from build123d import *

# Parameters (mm, degrees)
AUFSATZ_LINEAR_AUSTRAGEN1_DEPTH      = 43
AUFSATZ_LINEAR_AUSTRAGEN2_DEPTH      = 5
SCHNITT_LINEAR_AUSTRAGEN1_REACH      = 157.451
SKIZZE3_R                            = 1.5
SKIZZE4_W                            = 8
SKIZZE4_H                            = 16
SCHNITT_LINEAR_AUSTRAGEN2_DEPTH      = 18
SKIZZE5_W                            = 30
SKIZZE5_H                            = 39
SCHNITT_LINEAR_AUSTRAGEN3_DEPTH      = 18
SKIZZE6_W                            = 7
SKIZZE6_H                            = 7.5
SKIZZE6_H_2                          = 14
SKIZZE6_H_3                          = 5.5
AUFSATZ_LINEAR_AUSTRAGEN3_DEPTH      = 4
VERRUNDUNG1_R                        = 2
F_3_4_3_4_DURCHMESSER_BOHRUNG1_D     = 3.4
F_3_4_3_4_DURCHMESSER_BOHRUNG1_DEPTH = 4
SKIZZE10_W                           = 10
SKIZZE10_H                           = 33
SCHNITT_LINEAR_AUSTRAGEN4_DEPTH      = 1
SKIZZE11_W                           = 10
SKIZZE11_H                           = 33
SCHNITT_LINEAR_AUSTRAGEN5_DEPTH      = 0.1
SCHNITT_LINEAR_AUSTRAGEN7_DEPTH      = 39
SKIZZE15_W                           = 10.432594073
SKIZZE15_H                           = 24
SCHNITT_LINEAR_AUSTRAGEN10_DEPTH     = 16
SKIZZE16_W                           = 2.1
SKIZZE16_H                           = 39
SCHNITT_LINEAR_AUSTRAGEN11_DEPTH     = 2
VERRUNDUNG2_R                        = 20
VERRUNDUNG3_R                        = 10
SKIZZE17_W                           = 6
SKIZZE17_H                           = 6
AUFSATZ_LINEAR_AUSTRAGEN4_DEPTH      = 5
FASE1_SIZE                           = 6
F_3_4_3_4_DURCHMESSER_BOHRUNG2_D     = 3.4
F_3_4_3_4_DURCHMESSER_BOHRUNG2_DEPTH = 5
F_3_4_3_4_DURCHMESSER_BOHRUNG2_TIP   = 1.021463052


with BuildPart() as part:
    # Skizze1 → Aufsatz-Linear austragen1 (new body)
    with BuildSketch(Plane(origin=(0, 0, 0), x_dir=(1, 0, 0), z_dir=(0, 1, 0))):
        Polygon((0, 0), (50, 0), (78.641941074, 13.355956467), (70.189575839, 31.482112208), (34.843572145, 15), (0, 15), align=None)
    extrude(amount=AUFSATZ_LINEAR_AUSTRAGEN1_DEPTH)

    # Skizze2 → Aufsatz-Linear austragen2 (add)
    with BuildSketch(Plane(origin=(69.711631316, 0, -32.507067545), x_dir=(-0.4226182617407004, 0, -0.9063077870366495), z_dir=(0.9063077870366495, 0, -0.4226182617407004))):
        Polygon((-21.130913087, 43), (8.869086913, 43), (54.544231126, 88.675144213), (68.686366749, 74.533008589), (15.65335816, 21.5), (68.686366749, -31.533008589), (54.544231126, -45.675144213), (8.869086913, 0), (-21.130913087, 0), align=None)
    extrude(amount=AUFSATZ_LINEAR_AUSTRAGEN2_DEPTH)

    # Skizze3 → Schnitt-Linear austragen1 (cut, up to next)
    with BuildSketch(Plane.XY, mode=Mode.PRIVATE) as schnitt_linear_austragen1_sk1:
        with Locations((6, 39)):
            Circle(SKIZZE3_R)
    schnitt_linear_austragen1_tool1 = extrude(schnitt_linear_austragen1_sk1.sketch, amount=-SCHNITT_LINEAR_AUSTRAGEN1_REACH, mode=Mode.PRIVATE) & part.part
    # Skizze3 → Schnitt-Linear austragen1 (cut, up to next)
    with BuildSketch(Plane.XY, mode=Mode.PRIVATE) as schnitt_linear_austragen1_sk2:
        with Locations((20, 39)):
            Circle(SKIZZE3_R)
    schnitt_linear_austragen1_tool2 = extrude(schnitt_linear_austragen1_sk2.sketch, amount=-SCHNITT_LINEAR_AUSTRAGEN1_REACH, mode=Mode.PRIVATE) & part.part
    # Skizze3 → Schnitt-Linear austragen1 (cut, up to next)
    with BuildSketch(Plane.XY, mode=Mode.PRIVATE) as schnitt_linear_austragen1_sk3:
        with Locations((6, 4)):
            Circle(SKIZZE3_R)
    schnitt_linear_austragen1_tool3 = extrude(schnitt_linear_austragen1_sk3.sketch, amount=-SCHNITT_LINEAR_AUSTRAGEN1_REACH, mode=Mode.PRIVATE) & part.part
    # Skizze3 → Schnitt-Linear austragen1 (cut, up to next)
    with BuildSketch(Plane.XY, mode=Mode.PRIVATE) as schnitt_linear_austragen1_sk4:
        with Locations((20, 4)):
            Circle(SKIZZE3_R)
    schnitt_linear_austragen1_tool4 = extrude(schnitt_linear_austragen1_sk4.sketch, amount=-SCHNITT_LINEAR_AUSTRAGEN1_REACH, mode=Mode.PRIVATE) & part.part
    add(schnitt_linear_austragen1_tool1.solids().sort_by_distance((6, 39, 0))[0], mode=Mode.SUBTRACT)
    add(schnitt_linear_austragen1_tool2.solids().sort_by_distance((20, 39, 0))[0], mode=Mode.SUBTRACT)
    add(schnitt_linear_austragen1_tool3.solids().sort_by_distance((6, 4, 0))[0], mode=Mode.SUBTRACT)
    add(schnitt_linear_austragen1_tool4.solids().sort_by_distance((20, 4, 0))[0], mode=Mode.SUBTRACT)

    # Skizze4 → Schnitt-Linear austragen2 (cut)
    with BuildSketch(Plane.ZY):
        with Locations((-4, 21.5)):
            Rectangle(SKIZZE4_W, SKIZZE4_H)
    extrude(amount=-SCHNITT_LINEAR_AUSTRAGEN2_DEPTH, mode=Mode.SUBTRACT)

    # Skizze5 → Schnitt-Linear austragen3 (cut)
    with BuildSketch(Plane(origin=(0.477944523, 0, 1.024955337), x_dir=(-0.9063077870366492, 0, 0.4226182617407011), z_dir=(-0.4226182617407011, 0, -0.9063077870366492))):
        with Locations((-60.918274689, 21.5)):
            Rectangle(SKIZZE5_W, SKIZZE5_H)
    extrude(amount=-SCHNITT_LINEAR_AUSTRAGEN3_DEPTH, mode=Mode.SUBTRACT)

    # Skizze6 → Aufsatz-Linear austragen3 (add)
    with BuildSketch(Plane(origin=(8.085073234, 0, 17.338495504), x_dir=(-0.9063077870366492, 0, 0.42261826174070133), z_dir=(-0.42261826174070133, 0, -0.9063077870366492))):
        with Locations((-72.418274689, 37.25)):
            Rectangle(SKIZZE6_W, SKIZZE6_H)
        with Locations((-72.418274689, 18.5)):
            Rectangle(SKIZZE6_W, SKIZZE6_H_2)
        with Locations((-72.418274689, 4.75)):
            Rectangle(SKIZZE6_W, SKIZZE6_H_3)
    extrude(amount=AUFSATZ_LINEAR_AUSTRAGEN3_DEPTH)

    # Verrundung1
    verrundung1_edges = [part.edges().sort_by_distance(p)[0] for p in [
        (69.701005731, 33.5, -13.600241521),
        (69.701005731, 11.5, -13.600241521),
        (69.701005731, 25.5, -13.600241521),
        (69.701005731, 7.5, -13.600241521),
    ]]
    fillet(verrundung1_edges, radius=VERRUNDUNG1_R)

    # Ø3.4 (3.4) Durchmesser Bohrung1
    with Locations(Plane(origin=(6.394600187, 0, 13.713264356), x_dir=(-0.906307787036649, 0, 0.4226182617407016), z_dir=(-0.4226182617407016, 0, -0.906307787036649))):
        with Locations((-72.418274689, 37), (-72.418274689, 22), (-71.418274689, 14.1), (-71.418274689, 5)):
            Hole(F_3_4_3_4_DURCHMESSER_BOHRUNG1_D / 2, depth=F_3_4_3_4_DURCHMESSER_BOHRUNG1_DEPTH)

    # Skizze10 → Schnitt-Linear austragen4 (cut)
    with BuildSketch(Plane(origin=(8.085073234, 0, 17.338495504), x_dir=(-0.9063077870366492, 0, 0.42261826174070133), z_dir=(-0.42261826174070133, 0, -0.9063077870366492))):
        with Locations((-63.918274689, 21.5)):
            Rectangle(SKIZZE10_W, SKIZZE10_H)
    extrude(amount=-SCHNITT_LINEAR_AUSTRAGEN4_DEPTH, mode=Mode.SUBTRACT)

    # Skizze11 → Schnitt-Linear austragen5 (cut)
    with BuildSketch(Plane(origin=(8.930309758, 0, 19.151111078), x_dir=(0.9063077870366492, 0, -0.42261826174070133), z_dir=(0.42261826174070133, 0, 0.9063077870366492))):
        with Locations((63.918274689, 21.5)):
            Rectangle(SKIZZE11_W, SKIZZE11_H)
    extrude(amount=-SCHNITT_LINEAR_AUSTRAGEN5_DEPTH, mode=Mode.SUBTRACT)

    # Skizze12 → Schnitt-Linear austragen7 (cut)
    with BuildSketch(Plane(origin=(0, 2, 0), x_dir=(1, 0, 0), z_dir=(0, 1, 0))):
        Polygon((49.701163152, 2.067405927), (42.094034441, 18.380946094), (34.843572145, 15), (34.843572145, 12.5), (29.343572145, 12.5), (29.343572145, 2.067405927), align=None)
    extrude(amount=SCHNITT_LINEAR_AUSTRAGEN7_DEPTH, mode=Mode.SUBTRACT)

    # Skizze15 → Schnitt-Linear austragen10 (cut)
    with BuildSketch(Plane(origin=(29.343572145, 0, 0), x_dir=(0, 0, -1), z_dir=(1, 0, 0))):
        with Locations((7.283702963, 21.5)):
            Rectangle(SKIZZE15_W, SKIZZE15_H)
    extrude(amount=-SCHNITT_LINEAR_AUSTRAGEN10_DEPTH, mode=Mode.SUBTRACT)

    # Skizze16 → Schnitt-Linear austragen11 (cut)
    with BuildSketch(Plane(origin=(68.805323529, 0, -32.084449283), x_dir=(0.42261826174070133, 0, 0.9063077870366492), z_dir=(-0.9063077870366492, 0, 0.42261826174070133))):
        with Locations((2.180913087, 21.5)):
            Rectangle(SKIZZE16_W, SKIZZE16_H)
    extrude(amount=-SCHNITT_LINEAR_AUSTRAGEN11_DEPTH, mode=Mode.SUBTRACT)

    # Verrundung2
    verrundung2_edges = [part.edges().sort_by_distance(p)[0] for p in [
        (65.362005767, 21.5, -47.750373594),
    ]]
    fillet(verrundung2_edges, radius=VERRUNDUNG2_R)

    # Verrundung3
    verrundung3_edges = [part.edges().sort_by_distance(p)[0] for p in [
        (68.229162689, 43, -41.601735733),
        (68.229162689, 0, -41.601735733),
        (42.949287863, 74.533008589, -95.814602248),
        (48.926012637, 88.675144213, -82.997474607),
        (48.926012637, -45.675144213, -82.997474607),
        (42.949287863, -31.533008589, -95.814602248),
    ]]
    fillet(verrundung3_edges, radius=VERRUNDUNG3_R - 0.0001)  # a hair under: the kernel refuses the full size

    # Skizze17 → Aufsatz-Linear austragen4 (add)
    with BuildSketch(Plane(origin=(1.323181047, 0, 2.837570911), x_dir=(-0.9063077870366492, 0, 0.4226182617407011), z_dir=(-0.4226182617407011, 0, -0.9063077870366492))):
        with Locations((-40.918274689, 38)):
            Rectangle(SKIZZE17_W, SKIZZE17_H)
        with Locations((-40.918274689, 5)):
            Rectangle(SKIZZE17_W, SKIZZE17_H)
    extrude(amount=-AUFSATZ_LINEAR_AUSTRAGEN4_DEPTH)

    # Fase1
    fase1_edges = [part.edges().sort_by_distance(p)[0] for p in [
        (40.520823338, 2, -9.923700276),
        (40.520823338, 41, -9.923700276),
    ]]
    chamfer(fase1_edges, length=FASE1_SIZE - 0.0001)  # a hair under: the kernel refuses the full size

    # Ø3.4 (3.4) Durchmesser Bohrung2
    with Locations(Plane(origin=(1.323181047, 0, 2.837570911), x_dir=(-0.9063077870366492, 0, 0.4226182617407014), z_dir=(-0.42261826174070133, 0, -0.906307787036649))):
        with Locations((-40.918274689, 38), (-40.918274689, 5)):
            Hole(F_3_4_3_4_DURCHMESSER_BOHRUNG2_D / 2, depth=F_3_4_3_4_DURCHMESSER_BOHRUNG2_DEPTH)
            with Locations((0, 0, -(F_3_4_3_4_DURCHMESSER_BOHRUNG2_DEPTH + F_3_4_3_4_DURCHMESSER_BOHRUNG2_TIP / 2))):  # 118° drill point
                Cone(0, F_3_4_3_4_DURCHMESSER_BOHRUNG2_D / 2, F_3_4_3_4_DURCHMESSER_BOHRUNG2_TIP, mode=Mode.SUBTRACT)


solid = part.part
Geometry check sheet. Reference: the model listing, model coordinates, mm. A direction names the side the tool comes from. Round coordinates to 2 decimals unless told otherwise and drop trailing zeros. Write each loop counter-clockwise with the first axis right and the second up, starting at its lowest first coordinate (ties: lowest second). Pieces come first, ordered by that corner, then holes.
Item 1: Section check C-C (y = -10). Record the boundary of the cut face in (x, z).
Determined:
outline: (49.78, -75.24) - (54.32, -77.36) - (66.27, -51.72) - (61.74, -49.61) - close
Item 2: Mould release check, pull along Y, two halves, no side actions. Record for faces 1 (the face through (13.344, 21.7, -8.4)), 2 (the face through (68.373, 43.782, -41.377)), 3 (the face through (0, 21, -9)): +Y half, -Y half, draft (parallel to the pull), parting line (faces both ways), or undercut.
Determined:
face 1: undercut
face 2: +Y half
face 3: draft
Item 3: Access from +Z, -Z, +X, -X, +Y, -Y to the whole of each face (thin tool, end or side, straight path). Record for faces 4 (the face through (52.764, 0.986, -23.356)), 5 (the face through (7, 13.5, -4)), 6 (the face through (39, 35, -12)), 7 (the face through (72.777, 4.177, -17.241)), 8 (the face through (72.07, 18.6, -16.91)).
Determined:
face 4: -X, +Y, -Y
face 5: +Z, -X
face 6: -Z
face 7: none
face 8: -X
Item 4: Section check A-A (x = 20). Record the boundary of the cut face in (y, z).
Determined:
outline: (0, -15) - (2.5, -15) - (2.5, 0) - (0, 0) - close; (5.5, -15) - (37.5, -15) - (37.5, 0) - (5.5, 0) - close; (40.5, -15) - (43, -15) - (43, 0) - (40.5, 0) - close; hole (9.5, -12.5) - (33.5, -12.5) - (33.5, -2.07) - (9.5, -2.07) - close
Item 5: Go/stop test with flat-tipped pins: pin 1 Ø19.5 at (x, z) = (23.5, -19.5) entering from -Y; pin 2 Ø1.5 at (y, z) = (37.5, -61) entering from +X; pin 3 Ø9 at (x, z) = (50, -16) entering from +Y; pin 4 Ø6 at (y, z) = (-2, -76) entering from -X. Record where each tip stops, or that it passes through.
Determined:
pin 1: stops at y = 0
pin 2: stops at x = 62.29
pin 3: stops at y = 43
pin 4: passes through
Item 6: Material ranges on line 1 along Y through (x, z) = (6, -6); line 2 along Y through (x, z) = (20, -8.5); line 3 along Y through (x, z) = (6, -9.25), recorded low to high.
Determined:
line 1: y = 0 to 2.5, 5.5 to 13.5, 29.5 to 37.5, 40.5 to 43
line 2: y = 0 to 2.5, 5.5 to 9.5, 33.5 to 37.5, 40.5 to 43
line 3: y = 0 to 2.5, 5.5 to 37.5, 40.5 to 43
Item 7: Section check B-B (z = -66). Record the boundary of the cut face in (x, y).
Determined:
outline: (54.09, -28.09) - (59.61, -25.75) - (59.61, 2.53) - (54.09, 0.2) - close; (54.09, 42.8) - (59.61, 40.47) - (59.61, 68.75) - (54.09, 71.09) - close
